Design review of the part shown in the three views and the two pictorial views. Dimensions are in mm from the part's minimum x, y and z. Round coordinates to 2 decimals unless told otherwise and drop trailing zeros. Write each loop counter-clockwise with the first axis right and the second up, starting at its lowest first coordinate (ties: lowest second). Pieces come first, ordered by that corner, then holes. Notation, with made-up numbers: (17.25, 85) - (67.25, 85) arc R6 cw to (67.25, 89) - close; hole circle Ø6 at (62, -4). An arc over 180 degrees is marked (long way). Use one line per item in the form item = value.
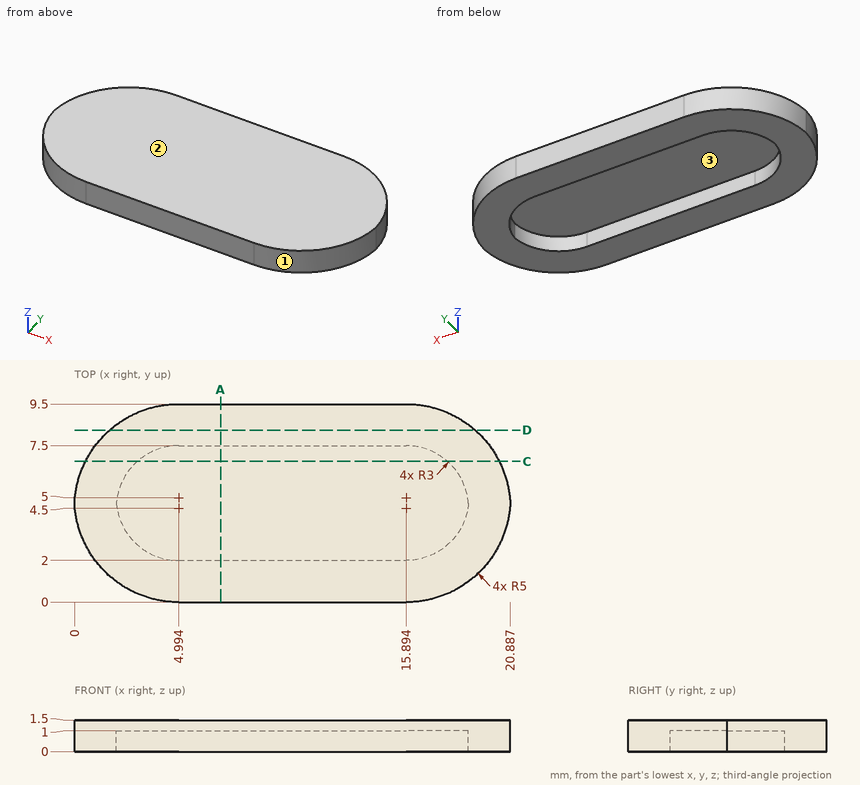
(1) Add section D-D on y = 8.25. Write out the cut boundary in (x, z).
Geometry results:
outline = (1.69, 0) - (19.2, 0) - (19.2, 1.5) - (1.69, 1.5) - close
(2) Insertion check: P1, Ø3, axis at x = 11, y = 4.5, coming from the -Z side; P2, Ø5, axis at x = 8.5, y = 7.5, coming from the -Z side. Each pin has a flat end and moves straight along its axis. Give the tip position at first contact, or say it passes through.
Geometry results:
P1 = 1
P2 = 0
(3) To check wall thickness, follow L1, parallel to Y at x = 10, z = 0.1; L2, parallel to X at y = 6, z = 0.2 (1 decimal); L3, parallel to Z at x = 10.5, y = 5. State the ranges of each line that lie inside material, in increasing order.
Geometry results:
L1 = 0 to 2, 7.5 to 9.5
L2 = 0.2 to 2.4, 18.5 to 20.7
L3 = 1 to 1.5
(4) The part is to be moulded in two halves that separate along X. For the marked faces 1, 2 and 3, say which applies: +X half, -X half, draft (parallel to the pull), parting line (faces both ways), or undercut.
Geometry results:
face_1 = +X half
face_2 = draft
face_3 = undercut
(5) Add section A-A on x = 7. Write out the cut boundary in (y, z).
Geometry results:
outline = (0, 0) - (2, 0) - (2, 1) - (7.5, 1) - (7.5, 0) - (9.5, 0) - (9.5, 1.5) - (0, 1.5) - close
(6) Add section C-C on y = 6.75. Write out the cut boundary in (x, z).
Geometry results:
outline = (0.53, 0) - (3.01, 0) - (3.01, 1) - (17.88, 1) - (17.88, 0) - (20.36, 0) - (20.36, 1.5) - (0.53, 1.5) - close
